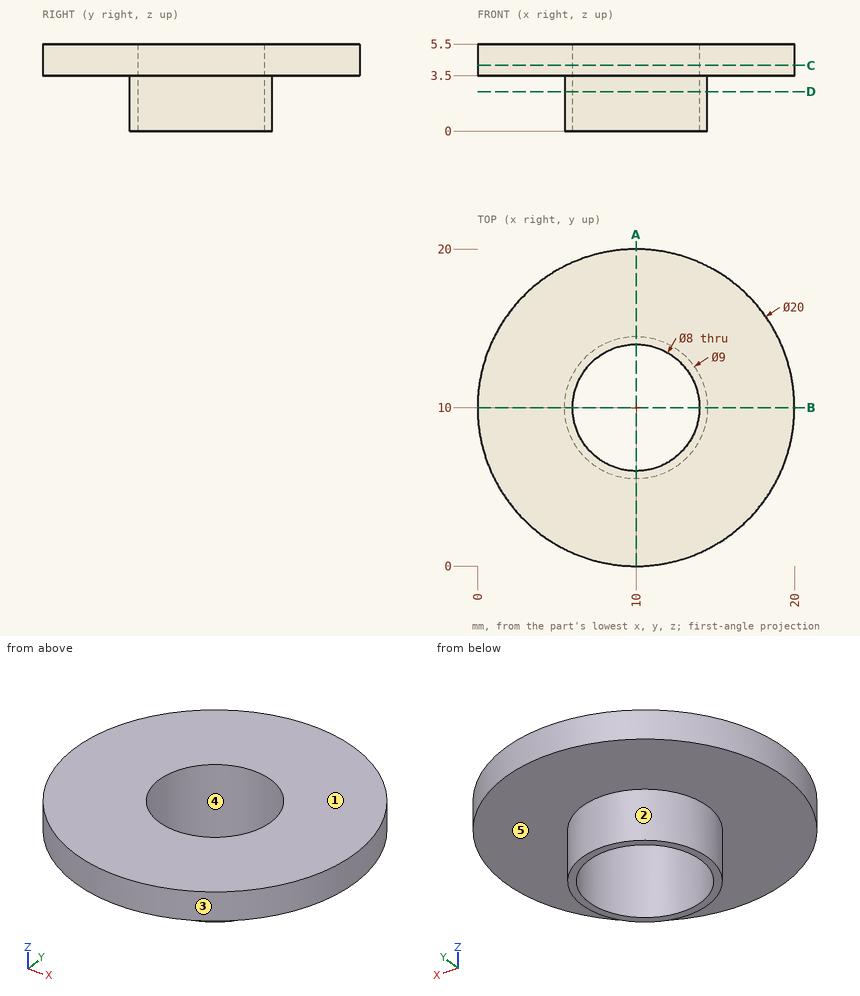
Verification items for this drawing (mm, ordinates from the low corner). A direction names the side the tool comes from. Give positions to 0.01 mm unless a question says otherwise; leave off trailing zeros. Write each loop counter-clockwise with the first axis right and the second up, starting at its lowest first coordinate (ties: lowest second). Pieces come first, ordered by that corner, then holes. Notation, with made-up numbers: (69, -35.75) - (73, -35.75) arc R33 ccw to (73, -2.75) - close; hole circle Ø10 at (42.5, 30). An arc over 180 degrees is marked (long way). Answer as a JSON object with one key per item and string values. Group by question number.
1) Depth check by flat-ended pin: P1, Ø3, axis at y = 14, z = 4.5, coming from the -X side; P2, Ø3, axis at y = 15, z = 5, coming from the -X side; P3, Ø2, axis at x = 4, z = 3.5, coming from the +Y side. Enter the tip coordinate at first touch or a pass-through.
2) Sectioned sample at A-A (x = 10). Record the cut outline in (y, z), then the cut area to 3 significant figures.
3) Access from +Z, -Z, +X, -X, +Y, -Y to the whole of each face (thin tool, end or side, straight path). Record for the marked faces 1 and 2.
4) Sectioned sample at C-C (z = 4.15). Record the cut outline in (x, y).
5) Thickness scan on probe 1 along Y at (x, z) = (10, 4.1); probe 2 along Y at (x, z) = (10, 1.9); probe 3 along Z at (x, y) = (6.5, 1). Record the ranges inside material, lowest first. Write a range as from..to.
6) Sectioned sample at D-D (z = 2.5). Record the cut outline in (x, y).
7) Release check for a two-part mould opening along X. For the marked faces 3, 4 and 5 record: pulls with the +X half, pulls with the -X half, needs draft (parallel to the pull), parting line crosses it, or undercut.
Geometry results:
{
 "1": {"P1": "stops at x = 0.32", "P2": "stops at x = 0.63", "P3": "stops at y = 18.66"},
 "2": {"outline": "(0, 3.5) - (5.5, 3.5) - (5.5, 0) - (6, 0) - (6, 5.5) - (0, 5.5) - close; (14, 0) - (14.5, 0) - (14.5, 3.5) - (20, 3.5) - (20, 5.5) - (14, 5.5) - close", "area": "27.5 mm^2"},
 "3": {"face 1": "+Z, +X, -X, +Y, -Y", "face 2": "-Z"},
 "4": {"outline": "circle Ø20 at (10, 10); hole circle Ø8 at (10, 10)"},
 "5": {"probe 1": "y = 0..6, 14..20", "probe 2": "y = 5.5..6, 14..14.5", "probe 3": "z = 3.5..5.5"},
 "6": {"outline": "circle Ø9 at (10, 10); hole circle Ø8 at (10, 10)"},
 "7": {"face 3": "parting line crosses it", "face 4": "undercut", "face 5": "needs draft"}
}
